Geometry check sheet. Reference: drawing and pictorial views, mm from the part's lowest x, y, z. Coordinates: 2 decimals unless noted, no trailing zeros. Loops run counter-clockwise (first coordinate to the right, second up) from the corner with the lowest first, then second, coordinate; pieces in that order, holes last. Notation, with made-up numbers: M -0.5,-6.75 L 57.5,-6.75 A31 cw 57.5,30.25 Z; hole C 2,53 d6. An arc over 180 degrees is marked long. Write each question's results on one line, items separated by ' | '. Start each with the question number.
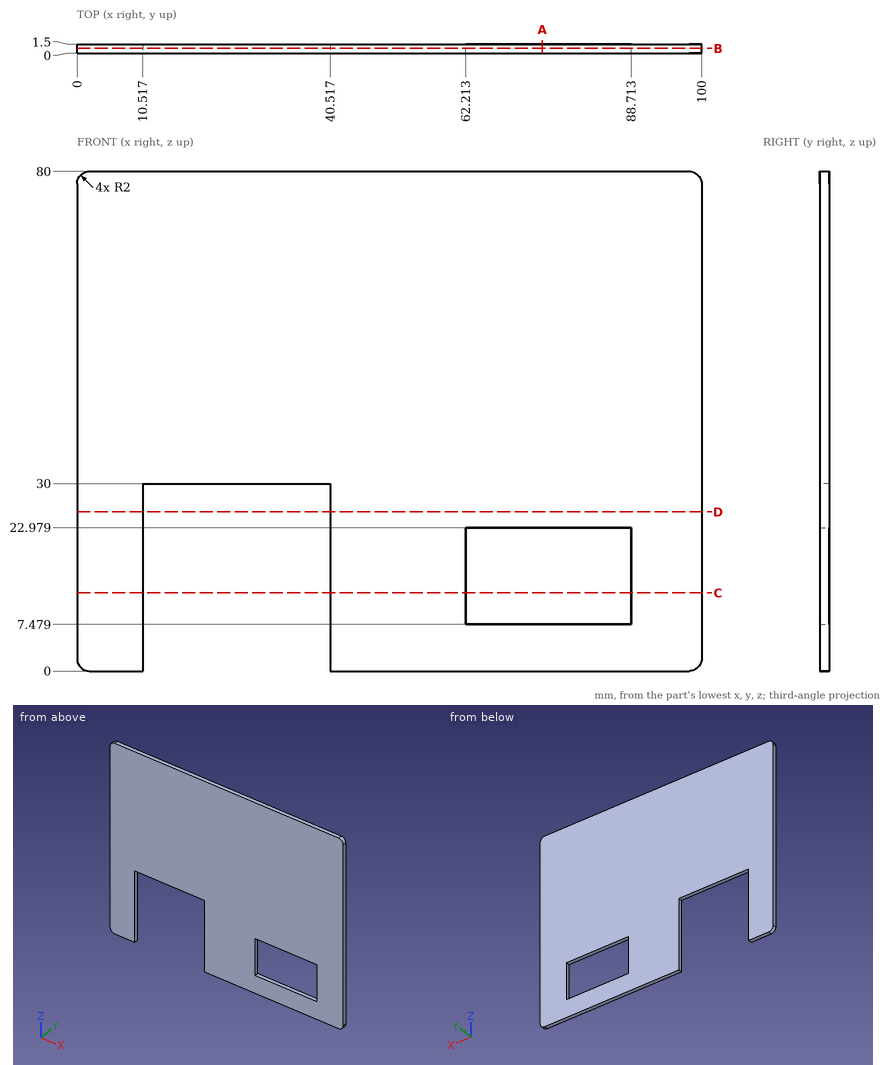
1) Section check C-C (z = 12.5). Enter the section's corners in (x, y).
2) Section check A-A (x = 74.5). Enter the section's corners in (y, z).
3) Thickness scan on probe 1 along Z at (x, y) = (62.5, 1); probe 2 along X at (y, z) = (0.3, 18); probe 3 along Z at (x, y) = (29, 1.05). Record the ranges inside material, lowest first.
4) Section check B-B (y = 0.8). Enter the section's corners in (x, z), then the cut area to 3 significant figures.
5) Section check D-D (z = 25.5). Enter the section's corners in (x, y).
Return value:
1) outline: M 0,0 L 10.52,0 L 10.52,1.5 L 0,1.5 Z; M 40.52,0 L 62.21,0 L 62.21,1.5 L 40.52,1.5 Z; M 88.71,0 L 100,0 L 100,1.5 L 88.71,1.5 Z
2) outline: M 0,0 L 1.5,0 L 1.5,7.48 L 0,7.48 Z; M 0,22.98 L 1.5,22.98 L 1.5,80 L 0,80 Z
3) probe 1: z = 0 to 7.48, 22.98 to 80 | probe 2: x = 0 to 10.52, 40.52 to 62.21, 88.71 to 100 | probe 3: z = 30 to 80
4) outline: M 0,2 A2 ccw 2,0 L 10.52,0 L 10.52,30 L 40.52,30 L 40.52,0 L 98,0 A2 ccw 100,2 L 100,78 A2 ccw 98,80 L 2,80 A2 ccw 0,78 Z; hole M 62.21,7.48 L 88.71,7.48 L 88.71,22.98 L 62.21,22.98 Z | area: 6,690 mm2
5) outline: M 0,0 L 10.52,0 L 10.52,1.5 L 0,1.5 Z; M 40.52,0 L 100,0 L 100,1.5 L 40.52,1.5 Z
